Design review of the part built by this model. Coordinates are the model's own, in mm. Face numbers are marked on the shaded views. A direction names the side the tool comes from. Round coordinates to 2 decimals unless told otherwise and drop trailing zeros. Order: outer loops, then holes, each group sorted by start corner. A loop starts at its lowest first (then second) coordinate and runs counter-clockwise, first axis right, second up. Notation, with made-up numbers: M -39.75,77.5 L 19.25,77.5 A9 ccw 19.25,89.5 Z; hole C -28.5,26.5 d1. An arc over 180 degrees is marked long. Use a Markdown table: item, result. Add a question column.
(1) Machinability: for the marked faces 4 and 5, which of the approach directions +Z, -Z, +X, -X, +Y, -Y give a long, thin tool a straight path to every point of the face, cutting with its end or side? Answer none if there is none.
(2) The part is to be moulded in two halves that separate along X. For the marked faces 1, 2 and 3, say which applies: released by +X, released by -X, zero draft, split by the parting line, or undercut.
(3) Take a section at C-C (x = 12). Write out the cut boundary in (y, z).
(4) Take a section at A-A (z = 0). Write out the cut boundary in (x, y), then the cut area to 3 significant figures.
(5) Take a section at B-B (y = 2). Write out the cut boundary in (x, z).
(6) To check wall thickness, follow probe 1 along X at (y, z) = (1.25, 0); probe 2 along X at (y, z) = (4.55, -3.75); probe 3 along X at (y, z) = (3.3, -0.5). State the ranges of each line that lie inside material, in increasing order. Write a range as from..to.
(7) For pin 1 (5 mm diameter, centred on x = -3.5, z = -6.5, fed in from +Y); pin 2 (3 mm diameter, centred on x = -12, z = 0, fed in from +Y), all flat-tipped, find the tip position at first contact; note any pin that passes through.
(8) Take a section at D-D (z = -9.5). Write out the cut boundary in (x, y).
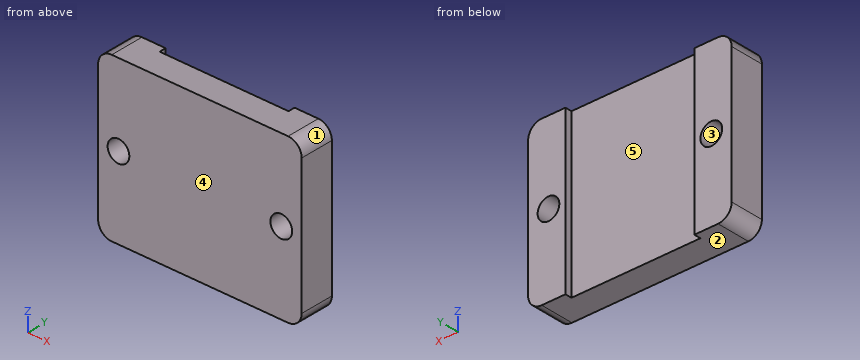
```python
from build123d import *

# Parameters (mm, degrees)
SKETCH_1_W      = 30
SKETCH_1_H      = 24
SKETCH_1_R      = 1.6
EXTRUDE_1_DEPTH = 4
SKETCH_2_W      = 5.5
SKETCH_2_H      = 24
SKETCH_2_R      = 1.6
EXTRUDE_2_DEPTH = 1
FILLET_1_R      = 2


with BuildPart() as part:
    # 草图1 → 凸台-拉伸1 (new body)
    with BuildSketch(Plane(origin=(0, 0, 0), x_dir=(1, 0, 0), z_dir=(0, 1, 0))):
        Rectangle(SKETCH_1_W, SKETCH_1_H)
        with Locations((-12, 0)):
            Circle(SKETCH_1_R, mode=Mode.SUBTRACT)
        with Locations((12, 0)):
            Circle(SKETCH_1_R, mode=Mode.SUBTRACT)
    extrude(amount=EXTRUDE_1_DEPTH)

    # 草图2 → 凸台-拉伸2 (add)
    with BuildSketch(Plane(origin=(0, 4, 0), x_dir=(1, 0, 0), z_dir=(0, 1, 0))):
        with Locations((-12.25, 0)):
            Rectangle(SKETCH_2_W, SKETCH_2_H)
        with Locations((-12, 0)):
            Circle(SKETCH_2_R, mode=Mode.SUBTRACT)
        with Locations((12.25, 0)):
            Rectangle(SKETCH_2_W, SKETCH_2_H)
        with Locations((12, 0)):
            Circle(SKETCH_2_R, mode=Mode.SUBTRACT)
    extrude(amount=EXTRUDE_2_DEPTH)

    # 圆角1
    fillet_1_edges = [part.edges().sort_by_distance(p)[0] for p in [
        (15, 2.5, 12),
        (-15, 2.5, 12),
        (-15, 2.5, -12),
        (15, 2.5, -12),
    ]]
    fillet(fillet_1_edges, radius=FILLET_1_R)


solid = part.part
```
Verdict:
| question | item | result |
|---|---|---|
| 1 | face 4 | +Z, -Z, +X, -X, -Y |
| 1 | face 5 | +Z, -Z, +Y |
| 2 | face 1 | released by +X |
| 2 | face 2 | zero draft |
| 2 | face 3 | undercut |
| 3 | outline | M 0,-12 L 5,-12 L 5,-1.6 L 0,-1.6 Z; M 0,1.6 L 5,1.6 L 5,12 L 0,12 Z |
| 4 | outline | M -15,0 L -13.6,0 L -13.6,5 L -15,5 Z; M -10.4,0 L 10.4,0 L 10.4,5 L 9.5,5 L 9.5,4 L -9.5,4 L -9.5,5 L -10.4,5 Z; M 13.6,0 L 15,0 L 15,5 L 13.6,5 Z |
| 4 | area | 99.0 mm^2 |
| 5 | outline | M -15,-10 A2 ccw -13,-12 L 13,-12 A2 ccw 15,-10 L 15,10 A2 ccw 13,12 L -13,12 A2 ccw -15,10 Z; hole C -12,0 d3.2; hole C 12,0 d3.2 |
| 6 | probe 1 | x = -15..-13.6, -10.4..10.4, 13.6..15 |
| 6 | probe 2 | x = -15..-9.5, 9.5..15 |
| 6 | probe 3 | x = -15..-13.52, -10.48..10.48, 13.52..15 |
| 7 | pin 1 | stops at y = 4 |
| 7 | pin 2 | passes through |
| 8 | outline | M -15,0 L 15,0 L 15,5 L 9.5,5 L 9.5,4 L -9.5,4 L -9.5,5 L -15,5 Z |
